```python
from build123d import *

# Parameters (mm, degrees)
BOSS_EXTRUDE1_DEPTH = 120
SKETCH4_R           = 3.3
CUT_EXTRUDE1_DEPTH  = 201.688813839


with BuildPart() as part:
    # Sketch2 → Boss-Extrude1 (new body)
    with BuildSketch(Plane.XY):
        Polygon((0, 0), (0, 100), (4, 100), (4, 4), (130, 4), (130, 0), align=None)
    extrude(amount=BOSS_EXTRUDE1_DEPTH)

    # Sketch4 → Cut-Extrude1 (cut, through all)
    with BuildSketch(Plane(origin=(4, 0, 0), x_dir=(0, 0, -1), z_dir=(1, 0, 0))):
        with Locations(Location((-100, 80, 0), (0, 0, 90))):
            Circle(SKETCH4_R)
        with Locations(Location((-20, 80, 0), (0, 0, 90))):
            Circle(SKETCH4_R)
        with Locations(Location((-20, 20, 0), (0, 0, 90))):
            Circle(SKETCH4_R)
        with Locations(Location((-100, 20, 0), (0, 0, 90))):
            Circle(SKETCH4_R)
    extrude(amount=-CUT_EXTRUDE1_DEPTH, mode=Mode.SUBTRACT)


solid = part.part
```
For this review, take the finished solid that the model builds, in its own axes (mm). A direction names the side the tool comes from. Coordinates: 2 decimals unless noted, no trailing zeros. Write each loop counter-clockwise with the first axis right and the second up, starting at its lowest first coordinate (ties: lowest second). Pieces come first, ordered by that corner, then holes. Notation, with made-up numbers: (-10, 27) - (16, 27) arc R32 ccw to (16, 57) - close; hole circle Ø5 at (9.5, 64). An arc over 180 degrees is marked (long way). Put each result on its own line as item: value.
1. Add section D-D, the plane x = 86. Give the boundary of the cut face in (y, z).
Values found:
outline: (0, 0) - (4, 0) - (4, 120) - (0, 120) - close
2. Add section C-C, the plane z = 85. Give the boundary of the cut face in (x, y), then the cut area to 3 significant figures.
Values found:
outline: (0, 0) - (130, 0) - (130, 4) - (4, 4) - (4, 100) - (0, 100) - close
area: 904 mm²
3. Mouldability with a two-part tool opening along Z and no side actions: class faces 1 (the flat face through (130, 2, 59)), 2 (the flat face through (36, 2, 0)), 3 (the cylindrical face through (2, 76.7, 20.1)), 4 (the cylindrical face through (2.03, 77.57, 102.23)) as released by +Z, released by -Z, zero draft, split by the parting line, or undercut.
Values found:
face 1: zero draft
face 2: released by -Z
face 3: undercut
face 4: undercut
4. Add section B-B, the plane y = 80. Give the boundary of the cut face in (x, z).
Values found:
outline: (0, 0) - (4, 0) - (4, 16.7) - (0, 16.7) - close; (0, 23.3) - (4, 23.3) - (4, 96.7) - (0, 96.7) - close; (0, 103.3) - (4, 103.3) - (4, 120) - (0, 120) - close
5. Add section A-A, the plane z = 100. Give the boundary of the cut face in (x, y), then the cut area to 3 significant figures.
Values found:
outline: (0, 0) - (130, 0) - (130, 4) - (4, 4) - (4, 16.7) - (0, 16.7) - close; (0, 23.3) - (4, 23.3) - (4, 76.7) - (0, 76.7) - close; (0, 83.3) - (4, 83.3) - (4, 100) - (0, 100) - close
area: 851 mm²
6. Machinability: for faces 5 (the flat face through (66, 0, 59)), 6 (the flat face through (66, 4, 59)), which of the approach directions +Z, -Z, +X, -X, +Y, -Y give a long, thin tool a straight path to every point of the face, cutting with its end or side? Answer none if there is none.
Values found:
face 5: +Z, -Z, +X, -X, -Y
face 6: +Z, -Z, +X, +Y
7. For pin 1 (2 mm diameter, centred on y = 65.5, z = 75, fed in from -X); pin 2 (2 mm diameter, centred on x = 85.5, z = 73.5, fed in from +Y); pin 3 (8.5 mm diameter, centred on y = 20, z = 20, fed in from +X); pin 4 (4 mm diameter, centred on y = 80, z = 100, fed in from +X), all flat-tipped, find the tip position at first contact; note any pin that passes through.
Values found:
pin 1: x = 0
pin 2: y = 4
pin 3: x = 4
pin 4: through
8. Wall thickness on probe 1 along Z at (x, y) = (1, 20); probe 2 along Y at (x, z) = (14, 41.5): over which ranges is each line inside the solid? List them lowest first.
Values found:
probe 1: 0 to 16.7, 23.3 to 96.7, 103.3 to 120
probe 2: 0 to 4
